Build history of the part. All positions in model axes, mm. A direction names the side the tool comes from. Round coordinates to 2 decimals unless told otherwise and drop trailing zeros. Write each loop counter-clockwise with the first axis right and the second up, starting at its lowest first coordinate (ties: lowest second). Pieces come first, ordered by that corner, then holes.
Item 1: Drop a flat-ended pin along its axis: pin 1 Ø6 at (y, z) = (-13.5, 4.5) entering from -X. Give the stop position or say it passes through.
Item 2: Mould opens along Z. For faces 3 (the flat face through (493, 0, -30)), 4 (the flat face through (493, -20, 0)), 5 (the flat face through (493, 0, -27)) say: +Z half, -Z half, draft (parallel to the pull), parting line (faces both ways), or undercut.
Item 3: Band-saw the part on B-B, the plane x = 215. Write the cut outline in (y, z), then the cut area to 3 significant figures.
Item 4: 3-axis set-ups, long thin cutter, end or side, ignore diameter. For faces 1 (the flat face through (1000, -18, 0)), 2 (the flat face through (493, 17, 0)): which of +Z, -Z, +X, -X, +Y, -Y reach the whole face in a straight line?
Item 5: Wall check: probe 1 along Z at (x, y) = (244, -3.5); probe 2 along Y at (x, z) = (756, 4); probe 3 along Z at (x, y) = (950, -18.3). Give the ranges that are in metal, low to high.
Item 6: Band-saw the part on A-A, the plane y = 10. Write the cut outline in (x, z).
```python
from build123d import *

# Parameters (mm, degrees)
SKETCH_1_W          = 54
SKETCH_1_H          = 34
EXTRUDE_1_DEPTH     = 1000
SKETCH_2_R          = 4.05
CUT_EXTRUDE_1_DEPTH = 41


with BuildPart() as part:
    # Эскиз1 → Вытянуть-Тонкостенный1 (new body)
    with BuildSketch(Plane(origin=(0, 0, 0), x_dir=(0, 0, -1), z_dir=(1, 0, 0))):
        with BuildLine():
            Line((30, 17), (30, -17))
            ThreePointArc((30, -17), (29.121320344, -19.121320344), (27, -20))
            Line((27, -20), (-27, -20))
            ThreePointArc((-27, -20), (-29.121320344, -19.121320344), (-30, -17))
            Line((-30, -17), (-30, 17))
            ThreePointArc((-30, 17), (-29.121320344, 19.121320344), (-27, 20))
            Line((-27, 20), (27, 20))
            ThreePointArc((27, 20), (29.121320344, 19.121320344), (30, 17))
        make_face()
        Rectangle(SKETCH_1_W, SKETCH_1_H, mode=Mode.SUBTRACT)
    extrude(amount=EXTRUDE_1_DEPTH)

    # Эскиз2 → Вырез-Вытянуть1 (cut, through all)
    with BuildSketch(Plane(origin=(0, 20, 0), x_dir=(1, 0, 0), z_dir=(0, 1, 0))):
        with Locations((950, -12)):
            Circle(SKETCH_2_R)
        with Locations((900, -12)):
            Circle(SKETCH_2_R)
        with Locations((850, -12)):
            Circle(SKETCH_2_R)
        with Locations((800, -12)):
            Circle(SKETCH_2_R)
        with Locations((650, -12)):
            Circle(SKETCH_2_R)
        with Locations((600, -12)):
            Circle(SKETCH_2_R)
        with Locations((550, -12)):
            Circle(SKETCH_2_R)
        with Locations((500, -12)):
            Circle(SKETCH_2_R)
    extrude(amount=-CUT_EXTRUDE_1_DEPTH, mode=Mode.SUBTRACT)


solid = part.part
```
Results:
1. pin 1: passes through
2. face 3: -Z half
2. face 4: draft
2. face 5: undercut
3. outline: (-20, -27) arc R3 ccw to (-17, -30) - (17, -30) arc R3 ccw to (20, -27) - (20, 27) arc R3 ccw to (17, 30) - (-17, 30) arc R3 ccw to (-20, 27) - close; hole (-17, -27) - (17, -27) - (17, 27) - (-17, 27) - close
3. area: 556 mm2
4. face 1: +Z, -Z, +X, +Y, -Y
4. face 2: +X, -X
5. probe 1: z = -30 to -27, 27 to 30
5. probe 2: y = -20 to -17, 17 to 20
5. probe 3: z = -29.7 to 7.95, 16.05 to 29.7
6. outline: (0, -30) - (1000, -30) - (1000, -27) - (0, -27) - close; (0, 27) - (1000, 27) - (1000, 30) - (0, 30) - close
